Geometry: see drawing. Coordinates: mm, zero at the bounding-box minimum. A direction names the side the tool comes from. Give positions to 0.01 mm unless a question says otherwise; leave off trailing zeros. Write each loop counter-clockwise with the first axis right and the second up, starting at its lowest first coordinate (ties: lowest second). Pieces come first, ordered by that corner, then holes. Notation, with made-up numbers: (10, 78.25) -> (26, 78.25) arc R9 ccw to (26, 84.25) -> close; hole circle Ø4 at (78, -30.75). An arc over 180 degrees is marked (long way). Answer as a JSON object with one key per item and string values. Group by question number.
Item 1: Section query A-A on y = 14. Return the cut outline in (x, z), plus the area to 3 significant figures.
Item 2: Pull-direction query (X, two-part tool) for the marked faces 3, 4 and 5; classes: pulls with the +X half, pulls with the -X half, needs draft (parallel to the pull), parting line crosses it, or undercut.
Item 3: First-contact query: pin 1 Ø2 at (y, z) = (19.5, 3) entering from -X; pin 2 Ø1.5 at (x, z) = (10.5, 6.5) entering from -Y; pin 3 Ø5 at (x, y) = (12, 25) entering from -Z. Flat tips, straight axial feed; report the tip coordinate or a pass-through.
Item 4: Section query D-D on y = 26.25. Return the cut outline in (x, z), plus the area to 3 significant figures.
Item 5: Access query for the marked faces 1 and 2. Directions: +Z, -Z, +X, -X, +Y, -Y. A direction counts if a zero-diameter tool reaches every point of the face in a straight line with its end or side. Return the directions, or none.
Item 6: Section query C-C on z = 17.75. Return the cut outline in (x, y).
Item 7: Ray query, probe 1 along X at (y, z) = (14, 6); probe 2 along X at (y, z) = (14, 17.5). Return the intervals inside material, ascending. Write a range as from..to.
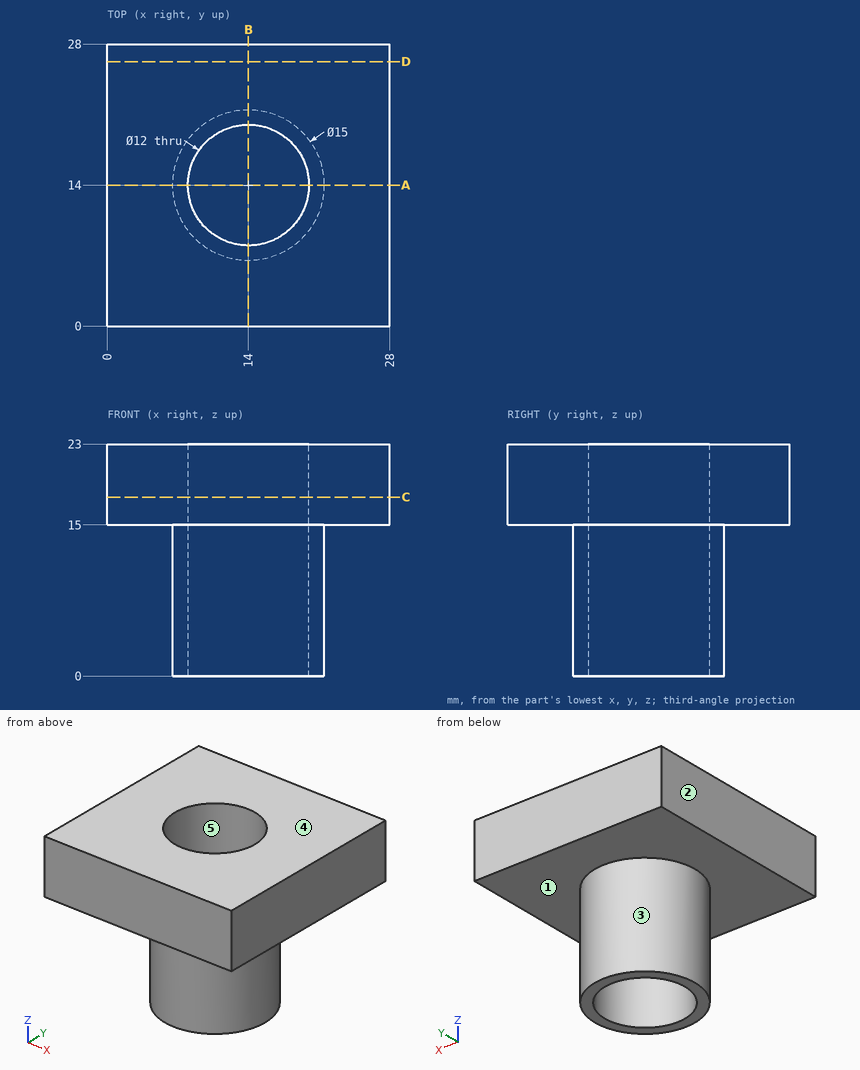
Worked answers:
{
 "1": {"outline": "(0, 15) -> (6.5, 15) -> (6.5, 0) -> (8, 0) -> (8, 23) -> (0, 23) -> close; (20, 0) -> (21.5, 0) -> (21.5, 15) -> (28, 15) -> (28, 23) -> (20, 23) -> close", "area": "173 mm^2"},
 "2": {"face 3": "parting line crosses it", "face 4": "needs draft", "face 5": "undercut"},
 "3": {"pin 1": "x = 8", "pin 2": "y = 7.02", "pin 3": "z = 15"},
 "4": {"outline": "(0, 15) -> (28, 15) -> (28, 23) -> (0, 23) -> close", "area": "224 mm^2"},
 "5": {"face 1": "-Z", "face 2": "+Z, -Z, -X, +Y, -Y"},
 "6": {"outline": "(0, 0) -> (28, 0) -> (28, 28) -> (0, 28) -> close; hole circle Ø12 at (14, 14)"},
 "7": {"probe 1": "6.5..8, 20..21.5", "probe 2": "0..8, 20..28"}
}
